Geometry check sheet. Reference: drawing and pictorial views, mm from the part's lowest x, y, z. A direction names the side the tool comes from. Round coordinates to 2 decimals unless told otherwise and drop trailing zeros. Loops run counter-clockwise (first coordinate to the right, second up) from the corner with the lowest first, then second, coordinate; pieces in that order, holes last. Notation, with made-up numbers: (-20.5, 54) - (31.5, 54) arc R20 cw to (31.5, 86) - close; hole circle Ø2 at (-28, 51). An arc over 180 degrees is marked (long way). Answer as CSV lines item,"result". Start each with the question number.
1) Cross-section at A-A on z = 30. Record the boundary of the cut face in (x, y).
2) Access from +Z, -Z, +X, -X, +Y, -Y to the whole of each face (thin tool, end or side, straight path). Record for the marked faces 1 and 2.
3) Depth check by flat-ended pin: P1, Ø12, axis at x = 9.5, z = 128, coming from the -Y side; P2, Ø16, axis at y = 10.5, z = 96.5, coming from the +X side; P3, Ø5, axis at x = 16, z = 85, coming from the -Y side. Enter the tip coordinate at first touch or a pass-through.
4) Thickness scan on line 1 along Y through (x, z) = (18.75, 18); line 2 along X through (y, z) = (9, 111). Record the ranges inside material, lowest first.
5) Cross-section at B-B on x = 17.75. Record the boundary of the cut face in (y, z), and give its area (3 significant figures).
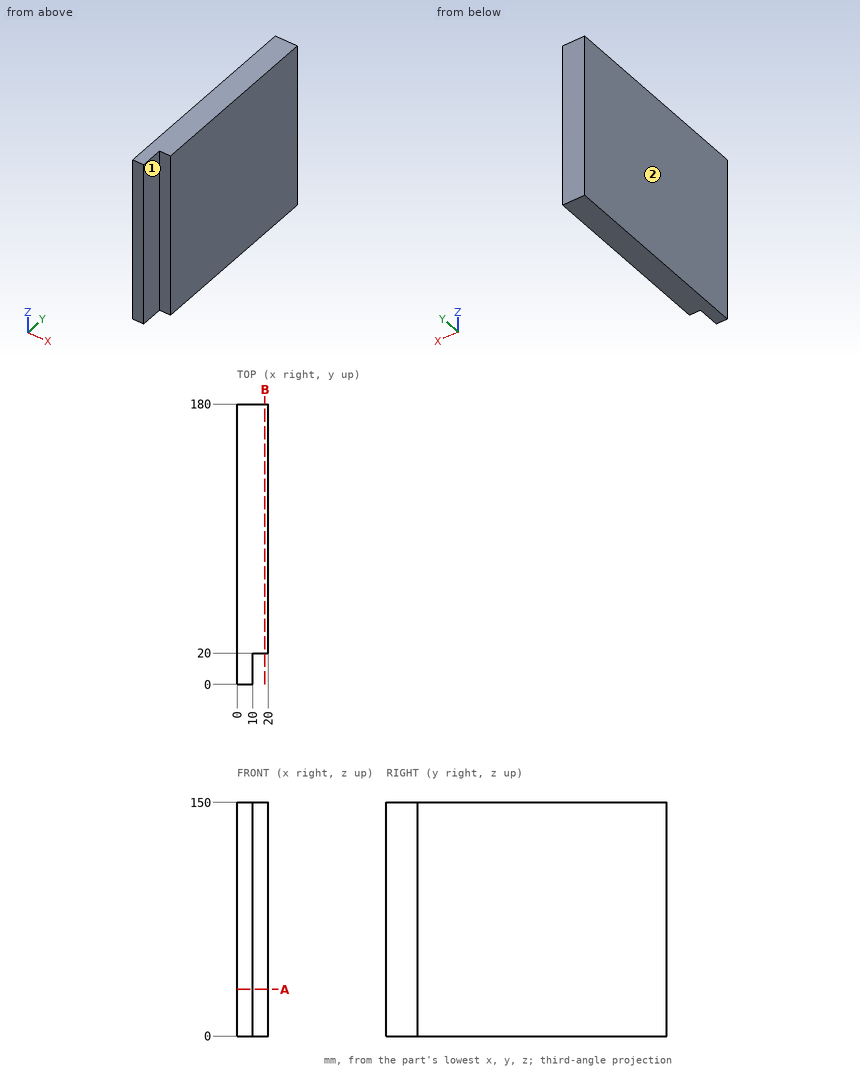
Answer block:
1,outline,"(0, 0) - (10, 0) - (10, 20) - (20, 20) - (20, 180) - (0, 180) - close"
2,face 1,"+Z, -Z, +X, -Y"
2,face 2,"+Z, -Z, -X, +Y, -Y"
3,P1,"stops at y = 0"
3,P2,"stops at x = 10"
3,P3,"stops at y = 20"
4,line 1,"y = 20 to 180"
4,line 2,"x = 0 to 10"
5,outline,"(20, 0) - (180, 0) - (180, 150) - (20, 150) - close"
5,area,"24,000 mm^2"
